Read the model definition and answer for the solid it produces. Units are mm, in the model's axes. A direction names the side the tool comes from. Round coordinates to 2 decimals unless told otherwise and drop trailing zeros. Order: outer loops, then holes, each group sorted by start corner. A loop starts at its lowest first (then second) coordinate and runs counter-clockwise, first axis right, second up. Notation, with made-up numbers: (-11.5, -30) - (46.5, -30) arc R9 ccw to (46.5, -25) - close; hole circle Ø4 at (-2, 39). An arc over 180 degrees is marked (long way). Answer as a JSON object with one key per item and string values. Group by question number.
Q1. A cutting plane is placed at B-B on x = -15. Determine the outline of the cut face in (y, z), and give its area (3 significant figures).
Q2. Consider line 1 (Z direction, x = 17, y = -19). Determine where the line is inside the solid, lowest interval first.
Q3. A cutting plane is placed at D-D on x = 17. Determine the outline of the cut face in (y, z).
Q4. A tool of negligible diameter and unlimited length cuts with its end or side. For faces 1 (the flat face through (-15, 0, 28)), 2 (the cylindrical face through (-19.77, -1.5, 23.7)), from which of +Z, -Z, +X, -X, +Y, -Y can it reach the whole face along a straight path? Write none if from no direction.
Q5. The mould has two halves that part along X. Classify faces 3 (the cylindrical face through (20.2, 2.4, 23.7)), 4 (the flat face through (0, 0, 0)), 5 (the flat face through (25, 0, 10)): pulls with the +X half, pulls with the -X half, needs draft (parallel to the pull), parting line crosses it, or undercut.
Q6. A cutting plane is placed at A-A on z = 25.25. Determine the outline of the cut face in (x, y).
Q7. A cutting plane is placed at C-C on y = 0. Determine the outline of the cut face in (x, z), and give its area (3 significant figures).
```python
from build123d import *

# Parameters (mm, degrees)
SKETCH_3_W      = 50
SKETCH_3_H      = 50
EXTRUDE_3_DEPTH = 20
SKETCH_4_R      = 5
SKETCH_4_R_2    = 4
EXTRUDE_4_DEPTH = 8
CHAMFER_2_SIZE  = 0.5
CHAMFER_3_SIZE  = 0.5


with BuildPart() as part:
    # 草图3 → 凸台-拉伸3 (new body)
    with BuildSketch(Plane.XY):
        Rectangle(SKETCH_3_W, SKETCH_3_H)
    extrude(amount=EXTRUDE_3_DEPTH)

    # 草图4 → 凸台-拉伸4 (add)
    with BuildSketch(Plane.XY.offset(20)):
        with Locations(Location((-15, 0, 0), (0, 0, 180))):
            Circle(SKETCH_4_R)
        with Locations(Location((17, 0, 0), (0, 0, 180))):
            Circle(SKETCH_4_R_2)
    extrude(amount=EXTRUDE_4_DEPTH)

    # 倒角2
    chamfer_2_edges = [part.edges().sort_by_distance(p)[0] for p in [
        (-10, 0, 28),
    ]]
    chamfer(chamfer_2_edges, length=CHAMFER_2_SIZE)

    # 倒角3
    chamfer_3_edges = [part.edges().sort_by_distance(p)[0] for p in [
        (21, 0, 28),
    ]]
    chamfer(chamfer_3_edges, length=CHAMFER_3_SIZE)


solid = part.part
```
Result set:
{
 "1": {"outline": "(-25, 0) - (25, 0) - (25, 20) - (5, 20) - (5, 27.5) - (4.5, 28) - (-4.5, 28) - (-5, 27.5) - (-5, 20) - (-25, 20) - close", "area": "1,080 mm²"},
 "2": {"line 1": "z = 0 to 20"},
 "3": {"outline": "(-25, 0) - (25, 0) - (25, 20) - (4, 20) - (4, 27.5) - (3.5, 28) - (-3.5, 28) - (-4, 27.5) - (-4, 20) - (-25, 20) - close"},
 "4": {"face 1": "+Z, +X, -X, +Y, -Y", "face 2": "+Z"},
 "5": {"face 3": "undercut", "face 4": "needs draft", "face 5": "pulls with the +X half"},
 "6": {"outline": "circle Ø10 at (-15, 0); circle Ø8 at (17, 0)"},
 "7": {"outline": "(-25, 0) - (25, 0) - (25, 20) - (21, 20) - (21, 27.5) - (20.5, 28) - (13.5, 28) - (13, 27.5) - (13, 20) - (-10, 20) - (-10, 27.5) - (-10.5, 28) - (-19.5, 28) - (-20, 27.5) - (-20, 20) - (-25, 20) - close", "area": "1,140 mm²"}
}
